Source: CAD feature listing. Evaluate the final solid. Frame: model axes, mm. A direction names the side the tool comes from. Give positions to 0.01 mm unless a question says otherwise; leave off trailing zeros. Order: outer loops, then holes, each group sorted by start corner. A loop starts at its lowest first (then second) coordinate and runs counter-clockwise, first axis right, second up. Notation, with made-up numbers: M 30.25,31.5 L 57.25,31.5 A23 cw 57.25,68.5 Z; hole C 24.5,74 d6. An arc over 180 degrees is marked long. Return JSON: item names as keys, results as strings.
from build123d import *

# Parameters (mm, degrees)
F0_W     = 101.6
F0_H     = 76.2
F1_DEPTH = 25.4
F4_R     = 5.08
F5_W     = 54.3147437274
F5_H     = 30.2147697657
F6_DEPTH = 14.2107922584


# Not quite as in the source:
# - the program builds the solid bodies; features that only make, move or delete a surface that nothing else refers to are left out


with BuildPart() as f1:
    # F0 (on Front) → F1 (new body)
    with BuildSketch(Plane.XZ):
        with Locations((-50.8, 38.1)):
            Rectangle(F0_W, F0_H)
    extrude(amount=F1_DEPTH)

    # F4
    f4_edges = [f1.edges().sort_by_distance(p)[0] for p in [
        (-101.6, -12.7, 76.2),
        (0, -12.7, 76.2),
        (0, -12.7, 0),
        (-101.6, -12.7, 0),
    ]]
    fillet(f4_edges, radius=F4_R)

    # F5 (on face) → F6 (join)
    with BuildSketch(Plane.XZ.offset(25.4)):
        with Locations((-58.2285393029, 24.9443138018)):
            Rectangle(F5_W, F5_H)
    extrude(amount=F6_DEPTH)


solid = f1.part
1. Section query D-D (x = -8). Return loops of the section in (y, z), then the cut area to 3 significant figures.
Evaluation:
{"outline": "M -25.4,0 L 0,0 L 0,76.2 L -25.4,76.2 Z", "area": "1,940 mm^2"}
2. Set-up query: faces 4 (the face through (-59, -32, 9.837)), 5 (the face through (-59, -32, 40.052)), 6 (the face through (-85.386, -32, 25)). Return all of +Z, -Z, +X, -X, +Y, -Y with unobstructed straight access to the full face (end or side cutting, diameter ignored); none if empty.
Evaluation:
{"face 4": "-Z, +X, -X, -Y", "face 5": "+Z, +X, -X, -Y", "face 6": "+Z, -Z, -X, -Y"}
3. Ray query, probe 1 along Y at (x, z) = (-16, 36); probe 2 along Z at (x, y) = (-47, -37); probe 3 along X at (y, z) = (-37, 24.5). Return the intervals inside material, ascending.
Evaluation:
{"probe 1": "y = -25.4 to 0", "probe 2": "z = 9.84 to 40.05", "probe 3": "x = -85.39 to -31.07"}
4. Draft query along X for faces 1 (the face through (0, -13, 38)), 2 (the face through (-52, -25.4, 47)), 3 (the face through (-101.6, -13, 38)). Return one class per face: pulls with the +X half, pulls with the -X half, needs draft (parallel to the pull), parting line crosses it, or undercut.
Evaluation:
{"face 1": "pulls with the +X half", "face 2": "needs draft", "face 3": "pulls with the -X half"}
5. Section query A-A (x = -72.5). Return loops of the section in (y, z).
Evaluation:
{"outline": "M -39.61,9.84 L -25.4,9.84 L -25.4,0 L 0,0 L 0,76.2 L -25.4,76.2 L -25.4,40.05 L -39.61,40.05 Z"}
6. First-contact query: pin 1 (1 mm diameter, centred on x = -57.5, z = 68, fed in from -Y); pin 2 (11.5 mm diameter, centred on y = -36, z = 25.5, fed in from -X); pin 3 (2 mm diameter, centred on x = -74.5, y = -28, fed in from +Z). Flat tips, straight axial feed; report the tip coordinate or a pass-through.
Evaluation:
{"pin 1": "stops at y = -25.4", "pin 2": "stops at x = -85.39", "pin 3": "stops at z = 40.05"}
7. Section query B-B (z = 12.5). Return loops of the section in (x, y), then the cut area to 3 significant figures.
Evaluation:
{"outline": "M -101.6,-25.4 L -85.39,-25.4 L -85.39,-39.61 L -31.07,-39.61 L -31.07,-25.4 L 0,-25.4 L 0,0 L -101.6,0 Z", "area": "3,350 mm^2"}
8. Section query C-C (y = -29). Return loops of the section in (x, z).
Evaluation:
{"outline": "M -85.39,9.84 L -31.07,9.84 L -31.07,40.05 L -85.39,40.05 Z"}
